Build history of the part. All positions in model axes, mm. A direction names the side the tool comes from. Coordinates: 2 decimals unless noted, no trailing zeros. Write each loop counter-clockwise with the first axis right and the second up, starting at its lowest first coordinate (ties: lowest second). Pieces come first, ordered by that corner, then holes. Notation, with made-up numbers: (54.25, 40) -> (66.25, 40) arc R26 cw to (66.25, 78) -> close; hole circle Ø3 at (85.5, 75). An arc over 180 degrees is marked (long way). Write each question's results on one line, items separated by ' | '. Start each with the question number.
Q1. Drop flat-ended pins along their axis: pin 1 Ø6 at (x, y) = (-29, 86) entering from -Z; pin 2 Ø2.5 at (x, y) = (-27.85, 83.87) entering from +Z. Give the stop position or say it passes through.
Q2. Two-plate mould, pull along X, no slides. Class faces 1 (the face through (-42.351, 84, 4)), 2 (the face through (-13.351, 84, 4)), 3 (the face through (-28, 69.371, 4)), 4 (the face through (-30, 85, 7)): released by +X, released by -X, zero draft, split by the parting line, or undercut.
Q3. Drill centre lines: line 1 (Y direction, x = -25, z = 4); line 2 (X direction, y = 84, z = 2.5); line 3 (Y direction, x = -28, z = 5.5). Where is each one in solid material? Low to high.
Q4. Saw through at C-C on y = 75.25. Give the cut face in (x, z), and give its area (3 significant figures).
Q5. Tool access for faces 5 (the face through (-40.851, 84, 2)), 6 (the face through (-26.669, 82.016, 7.493)): list every direction of +Z, -Z, +X, -X, +Y, -Y with a clear straight run to the whole face (end or side of a thin tool).
Q6. Saw through at A-A on x = -26.5. Give the cut face in (y, z), and give its area (3 significant figures).
Q7. Saw through at B-B on z = 3.75. Give the cut face in (x, y).
Q8. Saw through at D-D on x = -22. Give the cut face in (y, z).
from build123d import *

# Parameters (mm, degrees)
SKETCH002_W     = 29
SKETCH002_H     = 29
PAD001_DEPTH    = 8
SKETCH003_W     = 26
SKETCH003_H     = 26
POCKET001_DEPTH = 5
SKETCH004_W     = 6
SKETCH004_H     = 6
POCKET002_DEPTH = 2
SKETCH005_R     = 2.2
POCKET003_DEPTH = 5


with BuildPart() as part:
    # Sketch002 → Pad001 (new body)
    with BuildSketch(Plane.XY):
        with Locations((-27.851261, 83.870864)):
            Rectangle(SKETCH002_W, SKETCH002_H)
    extrude(amount=PAD001_DEPTH)

    # Sketch003 (on Face5 of Pad001) → Pocket001 (cut)
    with BuildSketch(Plane(origin=(0, 0, 0), x_dir=(1, 0, 0), z_dir=(0, 0, -1))):
        with Locations((-27.851261, -83.870864)):
            Rectangle(SKETCH003_W, SKETCH003_H)
    extrude(amount=-POCKET001_DEPTH, mode=Mode.SUBTRACT)

    # Sketch004 (on Face11 of Pocket001) → Pocket002 (cut)
    with BuildSketch(Plane(origin=(0, 0, 5), x_dir=(1, 0, 0), z_dir=(0, 0, -1))):
        with Locations((-27.851261, -83.870864)):
            Rectangle(SKETCH004_W, SKETCH004_H)
    extrude(amount=-POCKET002_DEPTH, mode=Mode.SUBTRACT)

    # Sketch005 (on Face16 of Pocket002) → Pocket003 (cut)
    with BuildSketch(Plane(origin=(0, 0, 7), x_dir=(1, 0, 0), z_dir=(0, 0, -1))):
        with Locations((-27.851261, -83.870864)):
            Circle(SKETCH005_R)
    extrude(amount=-POCKET003_DEPTH, mode=Mode.SUBTRACT)


solid = part.part
Returned:
1) pin 1: stops at z = 5 | pin 2: passes through
2) face 1: released by -X | face 2: released by +X | face 3: zero draft | face 4: undercut
3) line 1: y = 69.37 to 70.87, 96.87 to 98.37 | line 2: x = -42.35 to -40.85, -14.85 to -13.35 | line 3: y = 69.37 to 80.87, 86.87 to 98.37
4) outline: (-42.35, 0) -> (-40.85, 0) -> (-40.85, 5) -> (-14.85, 5) -> (-14.85, 0) -> (-13.35, 0) -> (-13.35, 8) -> (-42.35, 8) -> close | area: 102 mm2
5) face 5: -Z | face 6: +Z, -Z
6) outline: (69.37, 0) -> (70.87, 0) -> (70.87, 5) -> (80.87, 5) -> (80.87, 7) -> (82.13, 7) -> (82.13, 8) -> (69.37, 8) -> close; (85.61, 7) -> (86.87, 7) -> (86.87, 5) -> (96.87, 5) -> (96.87, 0) -> (98.37, 0) -> (98.37, 8) -> (85.61, 8) -> close | area: 86.5 mm2
7) outline: (-42.35, 69.37) -> (-13.35, 69.37) -> (-13.35, 98.37) -> (-42.35, 98.37) -> close; hole (-40.85, 70.87) -> (-14.85, 70.87) -> (-14.85, 96.87) -> (-40.85, 96.87) -> close
8) outline: (69.37, 0) -> (70.87, 0) -> (70.87, 5) -> (96.87, 5) -> (96.87, 0) -> (98.37, 0) -> (98.37, 8) -> (69.37, 8) -> close
